from build123d import *

# Parameters (mm, degrees)
BOSS_EXTRUDE1_DEPTH = 38.1
SKETCH2_R           = 12.065
CUT_EXTRUDE1_DEPTH  = 25.4
SKETCH7_R           = 12.065
CUT_EXTRUDE2_DEPTH  = 25.4
SKETCH9_W           = 26.289
SKETCH9_H           = 26.289
BOSS_EXTRUDE3_DEPTH = 8.89
SKETCH10_R          = 8.0645
CUT_EXTRUDE3_DEPTH  = 6.35
SKETCH12_R          = 6.35
CUT_EXTRUDE5_DEPTH  = 5.08
FILLET1_R           = 12.7
SKETCH13_R          = 1.35
CUT_EXTRUDE6_DEPTH  = 51.816


with BuildPart() as part:
    # Sketch1 → Boss-Extrude1 (new body)
    with BuildSketch(Plane(origin=(0, 0, 0), x_dir=(1, 0, 0), z_dir=(0, 1, 0))):
        with BuildLine():
            Line((-8.394951703, 35.720764917), (16.107614613, 27.828435078))
            ThreePointArc((16.107614613, 27.828435078), (18.03059142, 27.370657964), (20.001310729, 27.216823331))
            Line((20.001310729, 27.216823331), (122.238689271, 27.216823331))
            ThreePointArc((122.238689271, 27.216823331), (124.20940858, 27.370657964), (126.132385387, 27.828435078))
            Line((126.132385387, 27.828435078), (150.634951703, 35.720764917))
            ThreePointArc((150.634951703, 35.720764917), (157.509150211, 35.977683688), (163.508903941, 32.612632786))
            Line((163.508903941, 32.612632786), (184.96230509, 11.159231637))
            Line((184.96230509, 11.159231637), (158.021536726, -15.781536726))
            Line((158.021536726, -15.781536726), (142.24, 0))
            Line((142.24, 0), (127.676821583, 11.356327171))
            ThreePointArc((127.676821583, 11.356327171), (123.996342172, 13.351360126), (119.867179962, 14.041363479))
            Line((119.867179962, 14.041363479), (22.372820038, 14.041363479))
            ThreePointArc((22.372820038, 14.041363479), (18.243657828, 13.351360126), (14.563178417, 11.356327171))
            Line((14.563178417, 11.356327171), (0, 0))
            Line((0, 0), (-15.781536726, -15.781536726))
            Line((-15.781536726, -15.781536726), (-42.72230509, 11.159231637))
            Line((-42.72230509, 11.159231637), (-21.268903941, 32.612632786))
            ThreePointArc((-21.268903941, 32.612632786), (-15.269150211, 35.977683688), (-8.394951703, 35.720764917))
        make_face()
    extrude(amount=BOSS_EXTRUDE1_DEPTH)

    # Sketch2 → Cut-Extrude1 (cut)
    with BuildSketch(Plane(origin=(-15.781536726, 0, 15.781536726), x_dir=(0.7071067811865477, 0, 0.7071067811865475), z_dir=(-0.7071067811865475, 0, 0.7071067811865477))):
        with Locations((-19.05, 19.05)):
            Circle(SKETCH2_R)
    extrude(amount=-CUT_EXTRUDE1_DEPTH, mode=Mode.SUBTRACT)

    # Sketch7 → Cut-Extrude2 (cut)
    with BuildSketch(Plane(origin=(86.901536726, 0, 86.901536726), x_dir=(0.7071067811865472, 0, -0.7071067811865478), z_dir=(0.7071067811865478, 0, 0.7071067811865472))):
        with Locations((119.628868556, 19.05)):
            Circle(SKETCH7_R)
    extrude(amount=-CUT_EXTRUDE2_DEPTH, mode=Mode.SUBTRACT)

    # Sketch9 → Boss-Extrude3 (add)
    with BuildSketch(Plane(origin=(0, 0, -27.216823331), x_dir=(-1, 0, 0), z_dir=(0, 0, -1))):
        with Locations((-71.12, 13.1445)):
            Rectangle(SKETCH9_W, SKETCH9_H)
    extrude(amount=BOSS_EXTRUDE3_DEPTH)

    # Sketch10 → Cut-Extrude3 (cut)
    with BuildSketch(Plane(origin=(0, 0, -36.106823331), x_dir=(-1, 0, 0), z_dir=(0, 0, -1))):
        with Locations((-71.12, 13.1445)):
            Circle(SKETCH10_R)
    extrude(amount=-CUT_EXTRUDE3_DEPTH, mode=Mode.SUBTRACT)

    # Sketch12 → Cut-Extrude5 (cut)
    with BuildSketch(Plane(origin=(0, 0, -29.756823331), x_dir=(-1, 0, 0), z_dir=(0, 0, -1))):
        with Locations((-71.12, 13.1445)):
            Circle(SKETCH12_R)
    extrude(amount=-CUT_EXTRUDE5_DEPTH, mode=Mode.SUBTRACT)

    # Fillet1
    fillet1_edges = [part.edges().sort_by_distance(p)[0] for p in [
        (57.9755, 26.289, -31.661823331),
        (84.2645, 26.289, -31.661823331),
    ]]
    fillet(fillet1_edges, radius=FILLET1_R)

    # Sketch13 → Cut-Extrude6 (cut)
    with BuildSketch(Plane(origin=(0, 38.1, 0), x_dir=(1, 0, 0), z_dir=(0, 1, 0))):
        with Locations(Location((-15.525343469, 10.098073481, 0), (0, 0, 270))):
            Circle(SKETCH13_R)
        with Locations(Location((157.765343469, 10.098073481, 0), (0, 0, 270))):
            Circle(SKETCH13_R)
    extrude(amount=-CUT_EXTRUDE6_DEPTH, mode=Mode.SUBTRACT)


solid = part.part
CAD build for the part. Positions are in the model's coordinates, mm. A direction names the side the tool comes from. Coordinates: 2 decimals unless noted, no trailing zeros. Write each loop counter-clockwise with the first axis right and the second up, starting at its lowest first coordinate (ties: lowest second). Pieces come first, ordered by that corner, then holes. Notation, with made-up numbers: (-34, -6.5) - (20, -6.5) arc R32 ccw to (20, 28.5) - close; hole circle Ø2 at (71.5, -21). An arc over 180 degrees is marked (long way). Use a Markdown table: item, result. Add a question column.
Item 1: Band-saw the part on B-B, the plane x = 73.5. Give the cut face in (y, z).
Item 2: Band-saw the part on A-A, the plane y = 34. Give the cut face in (x, z), and give its area (3 significant figures).
Item 3: Band-saw the part on C-C, the plane x = 100. Give the cut face in (y, z), and give its area (3 significant figures).
Item 4: Drill centre lines: L1, parallel to X at y = 28, z = -9.5; L2, parallel to Z at x = 50, y = 16; L3, parallel to X at y = 12.5, z = -16. Where is each one in solid material? Low to high. Write a range as from..to.
Item 5: Mould opens along X. For faces 6 (the face through (-23.076, 10.317, 8.487)), 7 (the face through (73, 0, -16)), 8 (the face through (3.68, 18.78, -31.83)) say: pulls with the +X half, pulls with the -X half, needs draft (parallel to the pull), parting line crosses it, or undercut.
Item 6: Flat gauge pins, fed straight in: pin 1 (1.6 mm diameter, centred on x = -15.53, z = -10.1, fed in from -Y); pin 2 (10 mm diameter, centred on y = 7.5, z = -32, fed in from -X); pin 3 (4.5 mm diameter, centred on y = 8.5, z = -32, fed in from +X); pin 4 (2 mm diameter, centred on x = 124.5, y = 17, fed in from +Z). Where does each tip first touch, or does it go through?
Item 7: 3-axis set-ups, long thin cutter, end or side, ignore diameter. For faces 1 (the face through (79.177, 13.499, -32.976)), 2 (the face through (153.41, 19.22, -15.53)), 3 (the face through (18.003, 18.783, -27.375)), 4 (the face through (18.3, 18.78, -13.37)), 5 (the face through (-32.146, 18.783, -21.736)): which of +Z, -Z, +X, -X, +Y, -Y reach the whole face in a straight line?
Numbers:
| question | item | result |
|---|---|---|
| 1 | outline | (0, -36.11) - (5.44, -36.11) - (5.44, -29.76) - (7.26, -29.76) - (7.26, -24.68) - (19.03, -24.68) - (19.03, -29.76) - (20.85, -29.76) - (20.85, -36.11) - (26.14, -36.11) - (26.14, -27.22) - (38.1, -27.22) - (38.1, -14.04) - (0, -14.04) - close |
| 2 | outline | (-42.72, -11.16) - (-21.27, -32.61) arc R12.7 ccw to (-8.39, -35.72) - (16.11, -27.83) arc R12.7 cw to (20, -27.22) - (122.24, -27.22) arc R12.7 cw to (126.13, -27.83) - (150.63, -35.72) arc R12.7 ccw to (163.51, -32.61) - (184.96, -11.16) - (158.02, 15.78) - (142.24, 0) - (127.68, -11.36) arc R12.7 cw to (119.87, -14.04) - (22.37, -14.04) arc R12.7 cw to (14.56, -11.36) - (0, 0) - (-15.78, 15.78) - close; hole circle Ø2.7 at (-15.53, -10.1); hole circle Ø2.7 at (157.77, -10.1) |
| 2 | area | 5,030 mm2 |
| 3 | outline | (0, -27.22) - (38.1, -27.22) - (38.1, -14.04) - (0, -14.04) - close |
| 3 | area | 502 mm2 |
| 4 | L1 | -41.06..-28.88, -6..12.18, 130.06..148.24, 171.12..183.3 |
| 4 | L2 | -27.22..-14.04 |
| 4 | L3 | -37.88..-25.27, -11.64..153.88, 167.51..180.12 |
| 5 | face 6 | pulls with the -X half |
| 5 | face 7 | needs draft |
| 5 | face 8 | undercut |
| 6 | pin 1 | through |
| 6 | pin 2 | x = -26.88 |
| 6 | pin 3 | x = 166.37 |
| 6 | pin 4 | z = -12.72 |
| 7 | face 1 | -Z |
| 7 | face 2 | none |
| 7 | face 3 | -Z, +Y, -Y |
| 7 | face 4 | +Z, +Y, -Y |
| 7 | face 5 | -Z, -X, +Y, -Y |
